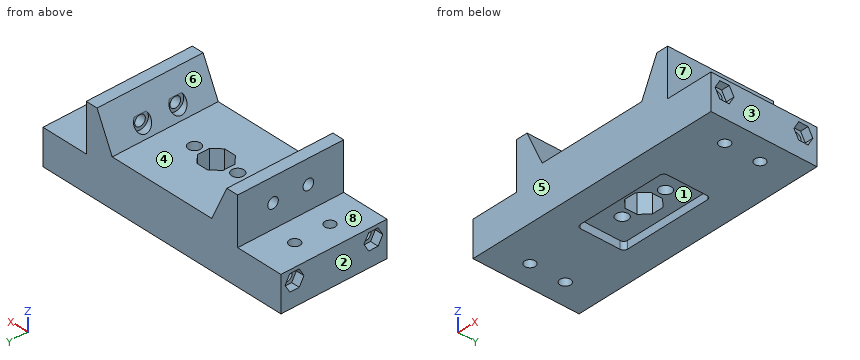
```python
from build123d import *

# Parameters (mm, degrees)
F0_W      = 110
F0_H      = 45
F1_DEPTH  = 15
F2_W      = 12
F2_H      = 45
F3_DEPTH  = 20
F4_R      = 2.25
F5_DEPTH  = 110.001
F6_R      = 2.25
F7_DEPTH  = 15.001
F8_R      = 2.25
F9_DEPTH  = 15.001
F10_R     = 3.55
F11_DEPTH = 3.5
F12_R     = 3.55
F13_DEPTH = 3.5
F3_FACE_W = 46
F3_FACE_H = 45
F14_DEPTH = 5
F16_DEPTH = 45.001
F17_R     = 2.55
F18_DEPTH = 35.001
F20_DEPTH = 3.3
F21_R     = 2.25
F22_DEPTH = 10
F24_DEPTH = 3.5
F25_R     = 2.25
F26_DEPTH = 10
F28_DEPTH = 3.5


with BuildPart() as f1:
    # F0 (on Top) → F1 (new body)
    with BuildSketch(Plane.XY):
        with Locations((55, 22.5)):
            Rectangle(F0_W, F0_H)
    extrude(amount=F1_DEPTH)

    # F2 (on face) → F3 (join)
    with BuildSketch(Plane.XY.offset(15)):
        with Locations((26, 22.5)):
            Rectangle(F2_W, F2_H)
        with Locations((84, 22.5)):
            Rectangle(F2_W, F2_H)
    extrude(amount=F3_DEPTH)

    # F4 (on Right) → F5 (cut, through all)
    with BuildSketch(Plane.YZ):
        with Locations((15, 25)):
            Circle(F4_R)
        with Locations((30, 25)):
            Circle(F4_R)
    extrude(amount=F5_DEPTH, mode=Mode.SUBTRACT)

    # F6 (on face) → F7 (cut, through all)
    with BuildSketch(Plane.XY.offset(15)):
        with Locations((10, 30)):
            Circle(F6_R)
        with Locations((10, 15)):
            Circle(F6_R)
    extrude(amount=-F7_DEPTH, mode=Mode.SUBTRACT)

    # F8 (on face) → F9 (cut, through all)
    with BuildSketch(Plane.XY.offset(15)):
        with Locations((100, 30)):
            Circle(F8_R)
        with Locations((100, 15)):
            Circle(F8_R)
    extrude(amount=-F9_DEPTH, mode=Mode.SUBTRACT)

    # F10 (on face) → F11 (cut)
    with BuildSketch(Plane(origin=(78, 0, 0), x_dir=(0, -1, 0), z_dir=(-1, 0, 0))):
        with Locations((-30, 25)):
            Circle(F10_R)
        with Locations((-15, 25)):
            Circle(F10_R)
    extrude(amount=-F11_DEPTH, mode=Mode.SUBTRACT)

    # F12 (on face) → F13 (cut)
    with BuildSketch(Plane.YZ.offset(32)):
        with Locations((15, 25)):
            Circle(F12_R)
        with Locations((30, 25)):
            Circle(F12_R)
    extrude(amount=-F13_DEPTH, mode=Mode.SUBTRACT)

    # F3_face (on face) → F14 (join)
    with BuildSketch(Plane(origin=(55, 22.5, 15), x_dir=(1, 0, 0), z_dir=(0, 0, 1))):
        Rectangle(F3_FACE_W, F3_FACE_H)
    extrude(amount=F14_DEPTH)

    # F15 (on face) → F16 (cut, through all)
    with BuildSketch(Plane.XZ):
        Polygon((32, 20), (32, 35), (25, 35), align=None)
        Polygon((85, 35), (78, 35), (78, 20), align=None)
    extrude(amount=-F16_DEPTH, mode=Mode.SUBTRACT)

    # F17 (on face) → F18 (cut, through all)
    with BuildSketch(Plane(origin=(0, 0, 0), x_dir=(1, 0, 0), z_dir=(0, 0, -1))):
        Polygon((57.5, -16.1), (55, -16.1), (52.5, -16.1), (49.1, -19.5), (49.1, -22), (49.1, -24.5), (52.5, -27.9), (55, -27.9), (57.5, -27.9), (60.9, -24.5), (60.9, -22), (60.9, -19.5), align=None)
        with Locations((45, -22)):
            Circle(F17_R)
        with Locations((65, -22)):
            Circle(F17_R)
    extrude(amount=-F18_DEPTH, mode=Mode.SUBTRACT)

    # F19 (on face) → F20 (cut)
    with BuildSketch(Plane(origin=(0, 0, 0), x_dir=(1, 0, 0), z_dir=(0, 0, -1))):
        with BuildLine():
            Line((73.45, -11.95), (55, -11.95))
            Line((55, -11.95), (36.55, -11.95))
            ThreePointArc((36.55, -11.95), (35.383274, -12.433274), (34.9, -13.6))
            Line((34.9, -13.6), (34.9, -30.4))
            ThreePointArc((34.9, -30.4), (35.383274, -31.566726), (36.55, -32.05))
            Line((36.55, -32.05), (73.45, -32.05))
            ThreePointArc((73.45, -32.05), (74.616726, -31.566726), (75.1, -30.4))
            Line((75.1, -30.4), (75.1, -13.6))
            ThreePointArc((75.1, -13.6), (74.616726, -12.433274), (73.45, -11.95))
        make_face()
    extrude(amount=-F20_DEPTH, mode=Mode.SUBTRACT)

    # F21 (on face) → F22 (cut)
    with BuildSketch(Plane(origin=(0, 0, 0), x_dir=(0, -1, 0), z_dir=(-1, 0, 0))):
        with Locations((-39.24, 10)):
            Circle(F21_R)
        with Locations((-5.76, 10)):
            Circle(F21_R)
    extrude(amount=-F22_DEPTH, mode=Mode.SUBTRACT)

    # F23 (on face) → F24 (cut)
    with BuildSketch(Plane(origin=(0, 0, 0), x_dir=(0, -1, 0), z_dir=(-1, 0, 0))):
        Polygon((-37.24, 13.5), (-39.24, 13.5), (-41.24, 13.5), (-43.24, 10), (-41.24, 6.5), (-39.24, 6.5), (-37.24, 6.5), (-35.24, 10), align=None)
        Polygon((-3.76, 13.5), (-5.76, 13.5), (-7.76, 13.5), (-9.76, 10), (-7.76, 6.5), (-5.76, 6.5), (-3.76, 6.5), (-1.76, 10), align=None)
    extrude(amount=-F24_DEPTH, mode=Mode.SUBTRACT)

    # F25 (on face) → F26 (cut)
    with BuildSketch(Plane.YZ.offset(110)):
        with Locations((5.76, 10)):
            Circle(F25_R)
        with Locations((39.24, 10)):
            Circle(F25_R)
    extrude(amount=-F26_DEPTH, mode=Mode.SUBTRACT)

    # F27 (on face) + F25 (on face) → F28 (cut)
    with BuildSketch(Plane.YZ.offset(110)):
        Polygon((7.76, 13.5), (5.76, 13.5), (3.76, 13.5), (1.76, 10), (3.76, 6.5), (5.76, 6.5), (7.76, 6.5), (9.76, 10), align=None)
        Polygon((37.24, 6.5), (39.24, 6.5), (41.24, 6.5), (43.24, 10), (41.24, 13.5), (39.24, 13.5), (37.24, 13.5), (35.24, 10), align=None)
    with BuildSketch(Plane.YZ.offset(110)):
        with Locations((5.76, 10)):
            Circle(F25_R)
        with Locations((39.24, 10)):
            Circle(F25_R)
    extrude(amount=-F28_DEPTH, mode=Mode.SUBTRACT)


solid = f1.part
```
Model file for the job. Use its own axes, mm. Face numbers are marked on the shaded views. A direction names the side the tool comes from. Round coordinates to 2 decimals unless told otherwise and drop trailing zeros. Write each loop counter-clockwise with the first axis right and the second up, starting at its lowest first coordinate (ties: lowest second). Pieces come first, ordered by that corner, then holes. Notation, with made-up numbers: (15.25, -29.75) - (71.25, -29.75) arc R11 ccw to (71.25, -16.75) - close; hole circle Ø1 at (4.5, 63). An arc over 180 degrees is marked (long way). Use CSV: the item, a comma, the result in double quotes. Start each with the question number.
Item 1: Band-saw the part on B-B (z = 18.5). Write the cut outline in (x, y).
Item 2: Band-saw the part on D-D (x = 65). Write the cut outline in (y, z).
Item 3: Band-saw the part on C-C (x = 53.5). Write the cut outline in (y, z), and give its area (3 significant figures).
Item 4: Band-saw the part on A-A (z = 30.5). Write the cut outline in (x, y).
Item 5: Two-plate mould, pull along X, no slides. Class the marked faces 1, 2, 3 and 4: released by +X, released by -X, zero draft, split by the parting line, or undercut.
Item 6: Drill centre lines: L1, parallel to Y at x = 87.25, z = 25; L2, parallel to Z at x = 7, y = 5.76; L3, parallel to Z at x = 63.5, y = 35. Where is each one in solid material? Low to high. Write a range as [from, to].
Item 7: Tool access for the marked faces 5, 6, 7 and 8: list every direction of +Z, -Z, +X, -X, +Y, -Y with a clear straight run to the whole face (end or side of a thin tool).
Item 8: Pin check, flat tips, straight feed: P1, Ø10, axis at x = 68, z = 27, coming from the +Y side; P2, Ø6, axis at y = 15, z = 25, coming from the -X side; P3, Ø9, axis at y = 15, z = 25, coming from the +X side; P4, Ø1.3, axis at y = 40, z = 10.5, coming from the -X side. Stop position of each tip, or through.
Checked values:
1,outline,"(20, 0) - (90, 0) - (90, 45) - (20, 45) - close; hole circle Ø5.1 at (45, 22); hole (49.1, 19.5) - (52.5, 16.1) - (57.5, 16.1) - (60.9, 19.5) - (60.9, 24.5) - (57.5, 27.9) - (52.5, 27.9) - (49.1, 24.5) - close; hole circle Ø5.1 at (65, 22)"
2,outline,"(0, 0) - (11.95, 0) - (11.95, 3.3) - (19.45, 3.3) - (19.45, 20) - (0, 20) - close; (24.55, 3.3) - (32.05, 3.3) - (32.05, 0) - (45, 0) - (45, 20) - (24.55, 20) - close"
3,outline,"(0, 0) - (11.95, 0) - (11.95, 3.3) - (16.1, 3.3) - (16.1, 20) - (0, 20) - close; (27.9, 3.3) - (32.05, 3.3) - (32.05, 0) - (45, 0) - (45, 20) - (27.9, 20) - close"
3,area,"637 mm²"
4,outline,"(20, 0) - (27.1, 0) - (27.1, 45) - (20, 45) - close; (82.9, 0) - (90, 0) - (90, 45) - (82.9, 45) - close"
5,face 1,"undercut"
5,face 2,"released by -X"
5,face 3,"released by +X"
5,face 4,"undercut"
6,L1,"y = [0, 12.75], [17.25, 27.75], [32.25, 45]"
6,L2,"z = [0, 7.75], [12.25, 15]"
6,L3,"z = [0, 20]"
7,face 5,"+Z, -Z, +X, -X, -Y"
7,face 6,"+Z, +Y, -Y"
7,face 7,"+Z, +X, +Y, -Y"
7,face 8,"+Z, -X, +Y, -Y"
8,P1,"passes through"
8,P2,"stops at x = 20"
8,P3,"stops at x = 90"
8,P4,"stops at x = 10"
